Drawing for the job (mm, zero at the part's lowest x, y, z). A direction names the side the tool comes from. Coordinates: 2 decimals unless noted, no trailing zeros. Loops run counter-clockwise (first coordinate to the right, second up) from the corner with the lowest first, then second, coordinate; pieces in that order, holes last. Notation, with made-up numbers: (10, 81.5) -> (25, 81.5) arc R19 ccw to (25, 110.5) -> close; hole circle Ø9 at (87, 55). An arc over 180 degrees is marked (long way). Write each question's results on one line, items separated by ' | '.
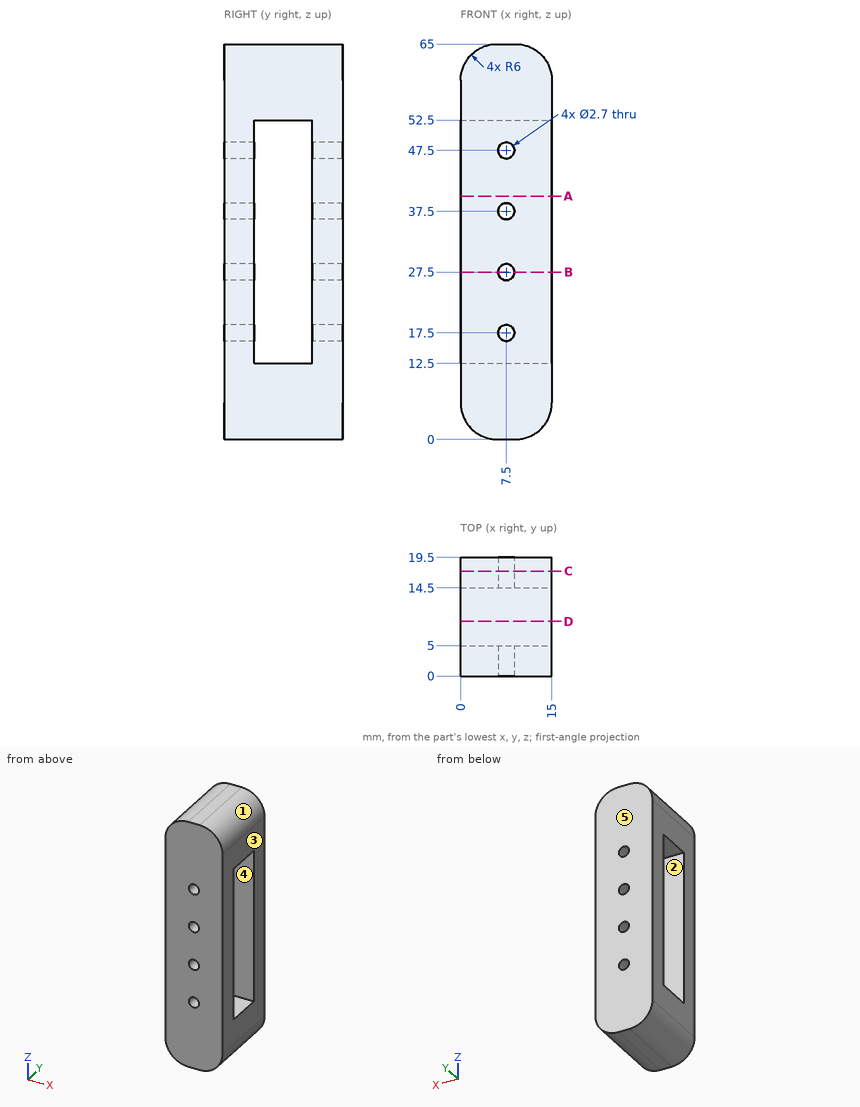
1) Which spindle directions (+Z, -Z, +X, -X, +Y, -Y) get a long thin tool onto all of the face, cutting with end or side? Do the marked faces 4 and 5. Say none if no direction does.
Outcome:
face 4: +X, -X | face 5: +Z, -Z, +X, -X, +Y
2) Slice it at A-A (z = 40). Write the cut outline in (x, y).
Outcome:
outline: (0, 0) -> (15, 0) -> (15, 5) -> (0, 5) -> close; (0, 14.5) -> (15, 14.5) -> (15, 19.5) -> (0, 19.5) -> close
3) Slice it at D-D (y = 9). Write the cut outline in (x, z).
Outcome:
outline: (0, 6) arc R6 ccw to (6, 0) -> (9, 0) arc R6 ccw to (15, 6) -> (15, 12.5) -> (0, 12.5) -> close; (0, 52.5) -> (15, 52.5) -> (15, 59) arc R6 ccw to (9, 65) -> (6, 65) arc R6 ccw to (0, 59) -> close
4) Slice it at B-B (z = 27.5). Write the cut outline in (x, y), then the cut area to 3 significant figures.
Outcome:
outline: (0, 0) -> (6.15, 0) -> (6.15, 5) -> (0, 5) -> close; (0, 14.5) -> (6.15, 14.5) -> (6.15, 19.5) -> (0, 19.5) -> close; (8.85, 0) -> (15, 0) -> (15, 5) -> (8.85, 5) -> close; (8.85, 14.5) -> (15, 14.5) -> (15, 19.5) -> (8.85, 19.5) -> close | area: 123 mm^2
5) Drill centre lines: L1, parallel to Z at x = 7.5, y = 1.45; L2, parallel to X at y = 16.85, z = 37.5; L3, parallel to Y at x = 1.75, z = 24.5. Where is each one in solid material? Low to high. Write a range as from..to.
Outcome:
L1: z = 0..16.15, 18.85..26.15, 28.85..36.15, 38.85..46.15, 48.85..65 | L2: x = 0..6.15, 8.85..15 | L3: y = 0..5, 14.5..19.5
6) Slice it at C-C (y = 17.25). Write the cut outline in (x, z), then the cut area to 3 significant figures.
Outcome:
outline: (0, 6) arc R6 ccw to (6, 0) -> (9, 0) arc R6 ccw to (15, 6) -> (15, 59) arc R6 ccw to (9, 65) -> (6, 65) arc R6 ccw to (0, 59) -> close; hole circle Ø2.7 at (7.5, 17.5); hole circle Ø2.7 at (7.5, 27.5); hole circle Ø2.7 at (7.5, 37.5); hole circle Ø2.7 at (7.5, 47.5) | area: 921 mm^2
7) Two-plate mould, pull along Z, no slides. Class the marked faces 1, 2 and 3: pulls with the +Z half, pulls with the -Z half, needs draft (parallel to the pull), parting line crosses it, or undercut.
Outcome:
face 1: pulls with the +Z half | face 2: undercut | face 3: needs draft
8) Pin check, flat tips, straight feed: pin 1 (3 mm diameter, centred on y = 12, z = 20.5, fed in from +X); pin 2 (5 mm diameter, centred on x = 12, y = 10, fed in from +Z). Stop position of each tip, or through.
Outcome:
pin 1: passes through | pin 2: stops at z = 64.98
